Verification items for the finished model (mm, model axes). A direction names the side the tool comes from. Round coordinates to 2 decimals unless told otherwise and drop trailing zeros. Order: outer loops, then holes, each group sorted by start corner. A loop starts at its lowest first (then second) coordinate and runs counter-clockwise, first axis right, second up.
```python
from build123d import *

# Parameters (mm, degrees)
CUT_EXTRUDE1_START = -12.700006
CUT_EXTRUDE1_DEPTH = 12.700012
CIRPATTERN1_COUNT  = 4


with BuildPart() as part:
    # Sketch1 → Revolve1 (revolve)
    with BuildSketch(Plane.XY):
        Polygon((0, 6.35), (0, 21.6662), (1.358992061, 25.4), (11.341007939, 25.4), (12.7, 21.6662), (12.7, 17.4625), (15.6718, 17.4625), (15.6718, 15.875), (19.7104, 15.875), (21.971, 17.4625), (30.48, 17.4625), (31.75, 16.1925), (31.75, 12.7), (37.3126, 12.7), (50.8, 9.83316463), (50.8, 7.9375), (38.1, 7.9375), (37.146133767, 6.35), align=None)
    revolve(axis=Axis((0, 0, 0), (1, 0, 0)))

    # Sketch2 → Cut-Extrude1 (cut)
    with BuildSketch(Plane.ZY.offset(CUT_EXTRUDE1_START)):
        with BuildLine():
            Line((-4.7625, 21.215720912), (-4.7625, 24.949520912))
            ThreePointArc((-4.7625, 24.949520912), (0, 25.4), (4.7625, 24.949520912))
            Line((4.7625, 24.949520912), (4.7625, 21.215720912))
            Line((4.7625, 21.215720912), (-4.7625, 21.215720912))
        make_face()
    cut_extrude1 = extrude(amount=CUT_EXTRUDE1_DEPTH, mode=Mode.SUBTRACT)

    # CirPattern1: Cut-Extrude1 ×4 about axis
    cirpattern1_axis = Axis((0, 0, 0), (1, 0, 0))
    for i in range(1, CIRPATTERN1_COUNT):
        add(cut_extrude1.rotate(cirpattern1_axis, i * 360 / CIRPATTERN1_COUNT), mode=Mode.SUBTRACT)


solid = part.part
```
1) Draft check along Z on faces 5 (the conical face through (0.236, -15.91, -15.646)), 6 (the flat face through (6, -23, 4.763)), 7 (the flat face through (6, -4.763, -23)), 8 (the cylindrical face through (6.42, 18.11, 17.81)). Enter one of: released by +Z, released by -Z, zero draft, split by the parting line, or undercut.
2) Scan lines: probe 1 along Z at (x, y) = (16, 0) (3 decimals); probe 2 along Z at (x, y) = (24, 0); probe 3 along X at (y, z) = (8.5, -12.5). Record each from-to range of solid material in increasing order.
3) Tool access check on faces 1 (the flat face through (6, -23, -4.762)), 2 (the flat face through (6, 4.762, -23)), 3 (the flat face through (15.672, 8, -14)), 4 (the flat face through (6, 23, 4.762)). Record the directions out of +Z, -Z, +X, -X, +Y, -Y that give a thin tool (end or side, any length) a straight path to the whole face; none if there is none.
4) Go/stop test with flat-tipped pins: pin 1 Ø1.5 at (x, z) = (7.5, 15) entering from +Y; pin 2 Ø3 at (x, y) = (3.5, 2) entering from +Z; pin 3 Ø1.9 at (x, z) = (6.5, 23) entering from -Y. Record where each tip stops, or that it passes through.
5) Sectioned sample at D-D on x = 21. Record the cut outline in (y, z).
Returned:
1. face 5: released by -Z
1. face 6: undercut
1. face 7: zero draft
1. face 8: released by +Z
2. probe 1: z = -15.875 to -6.35, 6.35 to 15.875
2. probe 2: z = -17.46 to -6.35, 6.35 to 17.46
2. probe 3: x = 0 to 31.75
3. face 1: +X, -X, -Y
3. face 2: -Z, +X, -X
3. face 3: none
3. face 4: +X, -X, +Y
4. pin 1: stops at y = 21.03
4. pin 2: stops at z = 21.22
4. pin 3: stops at y = -12.61
5. outline: circle Ø33.56 at (0, 0); hole circle Ø12.7 at (0, 0)
